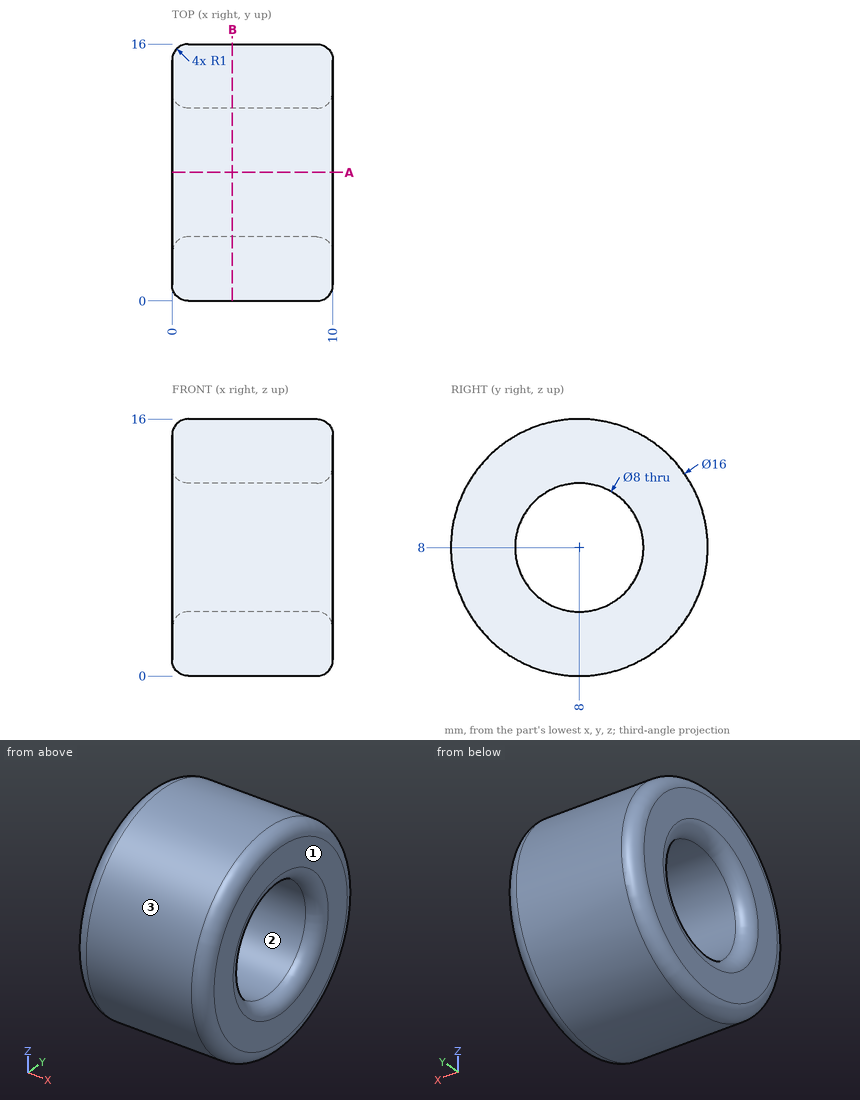
The figure shows three views and two pictorial views of one solid part (mm, origin at its lowest corner). Answer the questions. Round coordinates to 2 decimals unless told otherwise and drop trailing zeros. Write each loop counter-clockwise with the first axis right and the second up, starting at its lowest first coordinate (ties: lowest second). Pieces come first, ordered by that corner, then holes. Notation, with made-up numbers: M 19,-35.5 L 58,-35.5 A17 cw 58,-30.5 Z; hole C 25,-26 d2. An arc over 180 degrees is marked long. Use a Markdown table: item, result.
1) The part is cut by section B-B on x = 3.75. Give the vertices of the cut face in (y, z), plus the area to 3 significant figures.
Taken from the geometry:
| item | result |
|---|---|
| outline | C 8,8 d16; hole C 8,8 d8 |
| area | 151 mm2 |
2) Consider line 1 (Y direction, x = 5, z = 8); line 2 (X direction, y = 4.75, z = 1.75); line 3 (Y direction, x = 9.5, z = 9). Determine where each line is inside the solid, lowest interval first. Write a range as [from, to].
Taken from the geometry:
| item | result |
|---|---|
| line 1 | y = [0, 4], [12, 16] |
| line 2 | x = [0, 10] |
| line 3 | y = [0.2, 3.99], [12.01, 15.8] |
3) Determine the mould class of the marked faces 1, 2 and 3 for opening direction Y: pulls with the +Y half, pulls with the -Y half, needs draft (parallel to the pull), parting line crosses it, or undercut.
Taken from the geometry:
| item | result |
|---|---|
| face 1 | needs draft |
| face 2 | undercut |
| face 3 | parting line crosses it |
4) Flat-ended cylindrical pins translate along their axes: pin 1 (1.5 mm diameter, centred on x = 9, z = 6, fed in from +Y); pin 2 (1.5 mm diameter, centred on x = 3.5, y = 12, fed in from -Z); pin 3 (6 mm diameter, centred on x = 5.5, y = 4.5, fed in from +Z). Find the tip coordinate at first contact, or state that the pin passes through.
Taken from the geometry:
| item | result |
|---|---|
| pin 1 | stops at y = 15.9 |
| pin 2 | stops at z = 0.69 |
| pin 3 | stops at z = 15.98 |
5) The part is cut by section A-A on y = 8. Give the vertices of the cut face in (x, z).
Taken from the geometry:
| item | result |
|---|---|
| outline | M 0,1 A1 ccw 1,0 L 9,0 A1 ccw 10,1 L 10,3 A1 ccw 9,4 L 1,4 A1 ccw 0,3 Z; M 0,13 A1 ccw 1,12 L 9,12 A1 ccw 10,13 L 10,15 A1 ccw 9,16 L 1,16 A1 ccw 0,15 Z |
